```python
from build123d import *

# Parameters (mm, degrees)
SKETCH1_W           = 38.5
SKETCH1_H           = 29.5
BOSS_EXTRUDE1_DEPTH = 2
SKETCH2_W           = 13
SKETCH2_H           = 16
BOSS_EXTRUDE2_DEPTH = 4
SKETCH3_W           = 38.5
SKETCH3_H           = 4
BOSS_EXTRUDE3_DEPTH = 15
SKETCH4_R           = 1.65
CUT_EXTRUDE1_DEPTH  = 15
CUT_EXTRUDE2_DEPTH  = 2.5
SKETCH6_R           = 1.65
CUT_EXTRUDE3_DEPTH  = 2.5


with BuildPart() as part:
    # Sketch1 → Boss-Extrude1 (new body)
    with BuildSketch(Plane(origin=(0, 0, 0), x_dir=(1, 0, 0), z_dir=(0, 1, 0))):
        with Locations((19.25, -14.75)):
            Rectangle(SKETCH1_W, SKETCH1_H)
    extrude(amount=BOSS_EXTRUDE1_DEPTH)

    # Sketch2 → Boss-Extrude2 (add)
    with BuildSketch(Plane.XY.offset(29.5)):
        with Locations((19.25, -8)):
            Rectangle(SKETCH2_W, SKETCH2_H)
    extrude(amount=-BOSS_EXTRUDE2_DEPTH)

    # Sketch3 → Boss-Extrude3 (add)
    with BuildSketch(Plane.XZ):
        with Locations((19.25, 2)):
            Rectangle(SKETCH3_W, SKETCH3_H)
    extrude(amount=BOSS_EXTRUDE3_DEPTH)

    # Sketch4 → Cut-Extrude1 (cut)
    with BuildSketch(Plane.XY.offset(29.5)):
        with Locations((19.25, -4)):
            Circle(SKETCH4_R)
        with Locations((19.25, -12)):
            Circle(SKETCH4_R)
    extrude(amount=-CUT_EXTRUDE1_DEPTH, mode=Mode.SUBTRACT)

    # Sketch5 → Cut-Extrude2 (cut)
    with BuildSketch(Plane.XY.offset(4)):
        Polygon((11.732050808, -9), (13.464101615, -6), (11.732050808, -3), (8.267949192, -3), (6.535898385, -6), (8.267949192, -9), align=None)
        Polygon((30.232050808, -9), (31.964101615, -6), (30.232050808, -3), (26.767949192, -3), (25.035898385, -6), (26.767949192, -9), align=None)
    extrude(amount=-CUT_EXTRUDE2_DEPTH, mode=Mode.SUBTRACT)

    # Sketch6 → Cut-Extrude3 (cut)
    with BuildSketch(Plane.XY.offset(1.5)):
        with Locations((10, -6)):
            Circle(SKETCH6_R)
        with Locations((28.5, -6)):
            Circle(SKETCH6_R)
    extrude(amount=-CUT_EXTRUDE3_DEPTH, mode=Mode.SUBTRACT)


solid = part.part
```
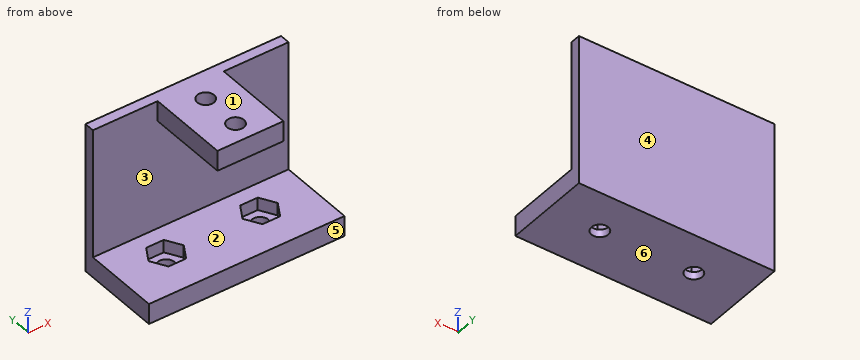
Source: CAD feature listing. Evaluate the final solid. Frame: model axes, mm. Face numbers are marked on the shaded views. A direction names the side the tool comes from. Coordinates: 2 decimals unless noted, no trailing zeros. Write each loop counter-clockwise with the first axis right and the second up, starting at its lowest first coordinate (ties: lowest second). Pieces come first, ordered by that corner, then holes. Notation, with made-up numbers: (-30, 49) - (2, 49) arc R9 ccw to (2, 57) - close; hole circle Ø3 at (-17, 52.5). An arc over 180 degrees is marked (long way). Answer as a JSON object with one key per item and string values.
Q1. First-contact query: pin 1 Ø2 at (x, y) = (10, -6) entering from +Z; pin 2 Ø7.5 at (x, y) = (26.5, -9.5) entering from +Z; pin 3 Ø3 at (x, z) = (18.5, 1.5) entering from -Y; pin 4 Ø4.5 at (y, z) = (-9, 28.5) entering from -X. Flat tips, straight axial feed; report the tip coordinate or a pass-through.
Ans:
{"pin 1": "passes through", "pin 2": "stops at z = 29.5", "pin 3": "stops at y = -15", "pin 4": "stops at x = 12.75"}
Q2. Section query D-D, the plane x = 19.25. Output: boundary loops of the cut face in (y, z).
Ans:
{"outline": "(-16, 25.5) - (-13.65, 25.5) - (-13.65, 29.5) - (-16, 29.5) - close; (-15, 0) - (2, 0) - (2, 29.5) - (-2.35, 29.5) - (-2.35, 25.5) - (0, 25.5) - (0, 4) - (-15, 4) - close; (-10.35, 25.5) - (-5.65, 25.5) - (-5.65, 29.5) - (-10.35, 29.5) - close"}
Q3. Set-up query: the marked faces 5 and 6. Return all of +Z, -Z, +X, -X, +Y, -Y with unobstructed straight access to the full face (end or side cutting, diameter ignored); none if empty.
Ans:
{"face 5": "-Z, +X, -X, -Y", "face 6": "-Z, +X, -X, +Y, -Y"}
Q4. Draft query along Z for the marked faces 1, 2, 3 and 4. Return one class per face: released by +Z, released by -Z, zero draft, split by the parting line, or undercut.
Ans:
{"face 1": "released by +Z", "face 2": "undercut", "face 3": "undercut", "face 4": "zero draft"}
Q5. Material intervals for line 1 (Y direction, x = 19.25, z = 26.8); line 2 (Y direction, x = 10, z = 0.85); line 3 (Z direction, x = 14.5, y = -14.5), sorted ascending. Write a range as [from, to].
Ans:
{"line 1": "y = [-16, -13.65], [-10.35, -5.65], [-2.35, 2]", "line 2": "y = [-15, -7.65], [-4.35, 2]", "line 3": "z = [0, 4], [25.5, 29.5]"}
Q6. Section query A-A, the plane y = -12. Output: boundary loops of the cut face in (x, z), plus the area to 3 significant figures.
Ans:
{"outline": "(0, 0) - (38.5, 0) - (38.5, 4) - (0, 4) - close; (12.75, 25.5) - (17.6, 25.5) - (17.6, 29.5) - (12.75, 29.5) - close; (20.9, 25.5) - (25.75, 25.5) - (25.75, 29.5) - (20.9, 29.5) - close", "area": "193 mm2"}
Q7. Section query B-B, the plane x = 10. Output: boundary loops of the cut face in (y, z), plus the area to 4 significant figures.
Ans:
{"outline": "(-15, 0) - (-7.65, 0) - (-7.65, 1.5) - (-9, 1.5) - (-9, 4) - (-15, 4) - close; (-4.35, 0) - (2, 0) - (2, 29.5) - (0, 29.5) - (0, 4) - (-3, 4) - (-3, 1.5) - (-4.35, 1.5) - close", "area": "99.05 mm2"}
Q8. Section query C-C, the plane z = 26. Output: boundary loops of the cut face in (x, y), plus the area to 3 significant figures.
Ans:
{"outline": "(0, 0) - (12.75, 0) - (12.75, -16) - (25.75, -16) - (25.75, 0) - (38.5, 0) - (38.5, 2) - (0, 2) - close; hole circle Ø3.3 at (19.25, -12); hole circle Ø3.3 at (19.25, -4)", "area": "268 mm2"}
